Autodesk Inventor part; units mm, degrees
ref_plane "YZ Plane" through (0, 0, 0) normal (1, 0, 0) x (0, 1, 0)
ref_plane "XZ Plane" through (0, 0, 0) normal (0, 1, 0) x (-1, 0, 0)
ref_plane "XY Plane" through (0, 0, 0) normal (0, 0, 1) x (1, 0, 0)
sketch "Sketch1" plane through (0, 0, 0) normal (0, 1, 0) x (-1, 0, 0)
  circle A0 centre (19.4253, 18.07) radius 1.05
  circle A1 centre (11.4453, 17) radius 1.05
  circle A2 centre (18.7453, 10) radius 1.05
  circle A3 centre (11.4453, 3) radius 1.05
  circle A4 centre (19.4253, 1.93) radius 1.05
  circle A5 centre (63.4253, 10) radius 2.6
  circle A6 centre (63.4253, 17) radius 1.05
  circle A7 centre (56.4253, 10) radius 1.05
  circle A8 centre (63.4253, 3) radius 1.05
  circle A9 centre (70.4253, 10) radius 1.05
  line L0 (10.3779, 20) -> (1.2846, 4.25)
  arc A10 (-0.694, 1.72) -> (1.2846, 4.25) centre (-8.6747, 10) ccw
  arc A11 (-0.694, 1.72) -> (0, 0) centre (0, 1) ccw
  line L1 (63.4253, 0) -> (0, 0)
  arc A12 (63.4253, 0) -> (63.4253, 20) centre (63.4253, 10) ccw
  line L2 (10.3779, 20) -> (63.4253, 20)
  point P0 (0, 0)
extrude "Extrusion1" add sketch "Sketch1" against normal blind 1.5
properties part number "CAM_axis_2_4_connector_frame_powered"
Could you check a few things on this model? Use its own coordinates, in mm. Give positions to 0.01 mm unless a question says otherwise; leave off trailing zeros. Loops run counter-clockwise (first coordinate to the right, second up) from the corner with the lowest first, then second, coordinate; pieces in that order, holes last. Notation, with made-up numbers: (80.25, -9) -> (122.25, -9) arc R27 cw to (122.25, 26) -> close; hole circle Ø1 at (83.5, 19.5). An arc over 180 degrees is marked (long way). Answer as CSV lines item,"result". Start each with the question number.
(1) If we section it at D-D on z = 14.25: Write out the boundary of the cut face in (x, y).
(2) If we section it at C-C on z = 5: Write out the boundary of the cut face in (x, y), then the cut area to 3 significant figures.
(3) We'd pull the mould along Z, two halves only. Please class faces 1 (the cylindrical face through (-61.36, -0.74, 8.42)), 2 (the flat face through (-36, 0, 10)), 3 (the cylindrical face through (-0.37, -0.74, 2.9)): released by +Z, released by -Z, zero draft, split by the parting line, or undercut.
(4) If we section it at A-A on y = -0.6: Count the separate pieces of the cut face and the enclosed holes in it, then the cut area to 3 significant figures.
(5) I need wall thicknesses on probe 1 along X at (y, z) = (-0.1, 9.25); probe 2 along Z at (x, y) = (-63.5, -0.4); probe 3 along X at (y, z) = (-0.3, 2.5). Which ranges of each line are inside material? Lowest first, please.
(6) If we section it at B-B on z = 10: Write out the boundary of the cut face in (x, y), then the cut area to 3 significant figures.
(7) I'm going to push a flat-ended pin straight in: pin 1 Ø4 at (x, z) = (-63.43, 10) entering from -Y. Where does the tip first touch, or does it pass through?
Computed:
1,outline,"(-72.48, -1.5) -> (-7.06, -1.5) -> (-7.06, 0) -> (-72.48, 0) -> close"
2,outline,"(-72.09, -1.5) -> (-1.72, -1.5) -> (-1.72, 0) -> (-72.09, 0) -> close"
2,area,"106 mm2"
3,face 1,"undercut"
3,face 2,"zero draft"
3,face 3,"released by +Z"
4,separate pieces,"1"
4,enclosed holes,"10"
4,area,"1,280 mm2"
5,probe 1,"x = -73.4 to -71.16, -69.69 to -65.91, -60.94 to -57.16, -55.69 to -19.48, -18.01 to -4.17"
5,probe 2,"z = 0 to 1.95, 4.05 to 7.4, 12.6 to 15.95, 18.05 to 20"
5,probe 3,"x = -70.04 to -64.35, -62.5 to -20.31, -18.54 to -12.37, -10.52 to -0.04"
6,outline,"(-73.43, -1.5) -> (-71.48, -1.5) -> (-71.48, 0) -> (-73.43, 0) -> close; (-69.38, -1.5) -> (-66.03, -1.5) -> (-66.03, 0) -> (-69.38, 0) -> close; (-60.83, -1.5) -> (-57.48, -1.5) -> (-57.48, 0) -> (-60.83, 0) -> close; (-55.38, -1.5) -> (-19.8, -1.5) -> (-19.8, 0) -> (-55.38, 0) -> close; (-17.7, -1.5) -> (-4.6, -1.5) -> (-4.6, 0) -> (-17.7, 0) -> close"
6,area,"86.0 mm2"
7,pin 1,"passes through"
